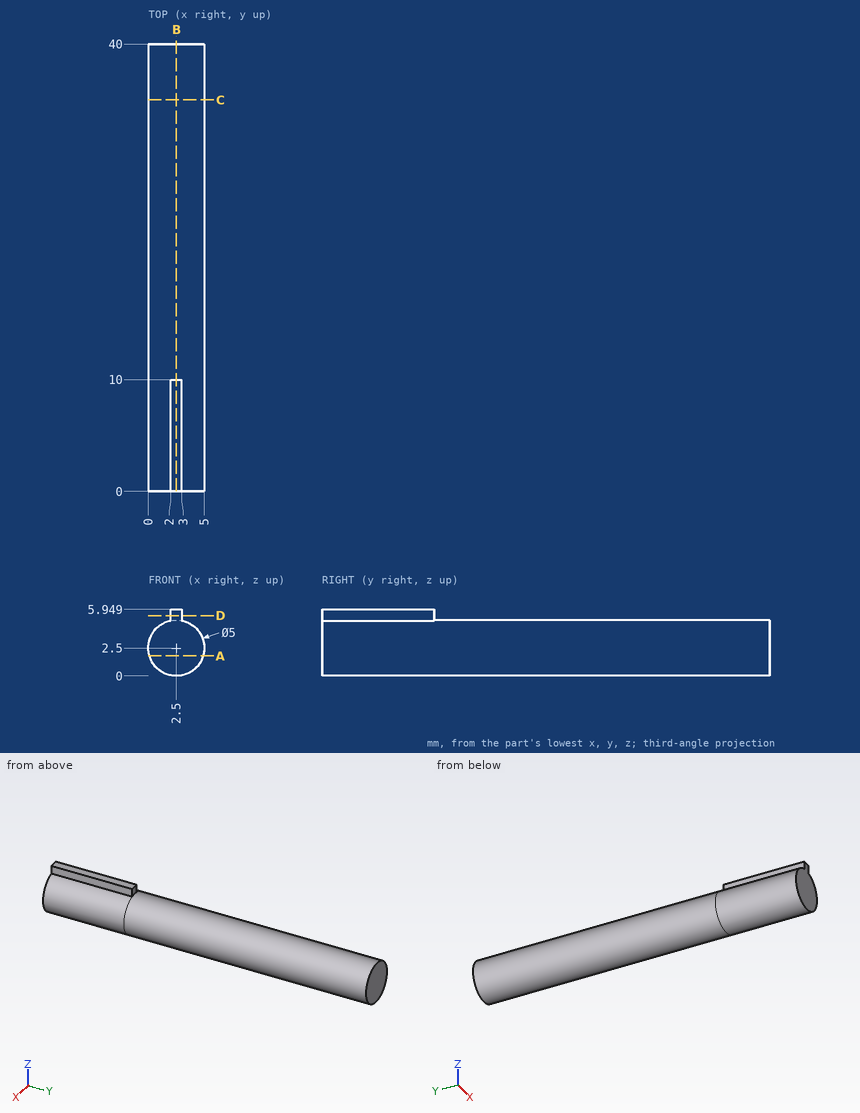
Here's the drawing with two shaded views (mm, measured from the low corner). I have some questions. Round coordinates to 2 decimals unless told otherwise and drop trailing zeros. Order: outer loops, then holes, each group sorted by start corner. A loop starts at its lowest first (then second) coordinate and runs counter-clockwise, first axis right, second up. Notation, with made-up numbers: (23, 60.5) -> (56, 60.5) arc R23 ccw to (56, 86.5) -> close; hole circle Ø2 at (-1, 51). An arc over 180 degrees is marked (long way). Return JSON: item names as keys, results as strings.
Q1. For pin 1 Ø0.5 at (y, z) = (6.5, 5.5) entering from +X; pin 2 Ø1.5 at (x, y) = (4.5, 13) entering from -Z (1 decimal), each with a flat end and sliding along its axis, tell me the tip position at first contact or that it passes through.
Filled sheet:
{"pin 1": "stops at x = 3", "pin 2": "stops at z = 0.3"}
Q2. If we section it at D-D on z = 5.4: List the corners of the cut face in (x, y) for me.
Filled sheet:
{"outline": "(2, 0) -> (3, 0) -> (3, 10) -> (2, 10) -> close"}
Q3. If we section it at C-C on y = 35: List the corners of the cut face in (x, z) for me.
Filled sheet:
{"outline": "circle Ø5 at (2.5, 2.5)"}
Q4. If we section it at B-B on x = 2.5: List the corners of the cut face in (y, z) for me.
Filled sheet:
{"outline": "(0, 0) -> (40, 0) -> (40, 5) -> (10, 5) -> (10, 5.95) -> (0, 5.95) -> close"}
Q5. If we section it at A-A on z = 1.8: List the corners of the cut face in (x, y) for me.
Filled sheet:
{"outline": "(0.1, 0) -> (4.9, 0) -> (4.9, 40) -> (0.1, 40) -> close"}
Q6. I need wall thicknesses on line 1 along X through (y, z) = (9, 2.6); line 2 along Z through (x, y) = (2.7, 20.5); line 3 along X through (y, z) = (17.5, 3.45). Which ranges of each line are inside material? Lowest first, please. Write a range as from..to.
Filled sheet:
{"line 1": "x = 0..5", "line 2": "z = 0.01..4.99", "line 3": "x = 0.19..4.81"}
